Here's how the part is built. I have some questions about the finished solid (model axes, mm). Face numbers are marked on the shaded views. A direction names the side the tool comes from. Round coordinates to 2 decimals unless told otherwise and drop trailing zeros. Order: outer loops, then holes, each group sorted by start corner. A loop starts at its lowest first (then second) coordinate and runs counter-clockwise, first axis right, second up.
```python
from build123d import *


with BuildPart() as part:
    # Sketch1 → Revolve1 (revolve)
    with BuildSketch(Plane(origin=(0, 0, 0), x_dir=(-1, 0, 0), z_dir=(0, 0, -1)), mode=Mode.PRIVATE) as revolve1_sk:
        with BuildLine():
            Line((-1.5, -30), (0, -30))
            Line((0, -30), (0, 0))
            Line((0, 0), (-2.7, 0))
            ThreePointArc((-2.7, 0), (-2.95, -0.25), (-2.7, -0.5))
            Line((-2.7, -0.5), (-2.25, -2))
            Line((-2.25, -2), (-2, -2))
            Line((-2, -2), (-2, -29.5))
            Line((-2, -29.5), (-1.5, -30))
        make_face()
    revolve(revolve1_sk.sketch.rotate(Axis((0, -30, 0), (0, 1, 0)), 270), axis=Axis((0, -30, 0), (0, 1, 0)))


solid = part.part
```
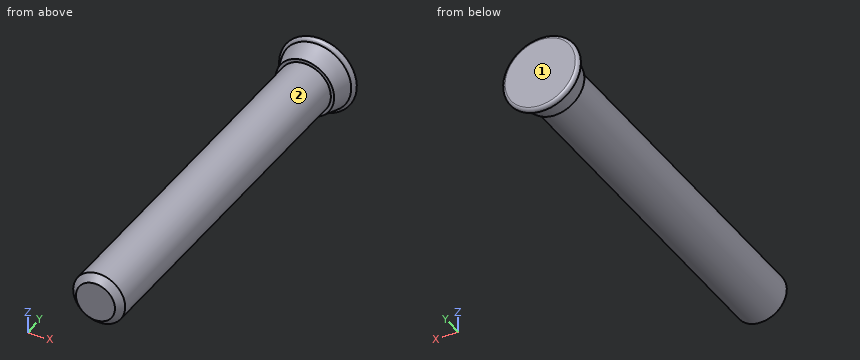
1. On a 3-axis mill with a long thin cutter (end or side, diameter ignored), from which of +Z, -Z, +X, -X, +Y, -Y can I reach the whole of each face in a straight line? I mean the marked faces 1 and 2. Say none if no direction works.
Evaluation:
face 1: +Z, -Z, +X, -X, +Y
face 2: -Y
2. I'm going to push flat-ended pins straight in: P1, Ø2, axis at y = -25.5, z = -1.5, coming from the -X side; P2, Ø1.5, axis at x = 1, y = -9.5, coming from the +Z side. Where does each tip first touch, or does it pass through?
Evaluation:
P1: stops at x = -1.94
P2: stops at z = 1.98
3. If we section it at B-B, the plane z = 0: Write out the boundary of the cut face in (x, y).
Evaluation:
outline: (-2.7, -0.5) - (-2.25, -2) - (-2, -2) - (-2, -29.5) - (-1.5, -30) - (1.5, -30) - (2, -29.5) - (2, -2) - (2.25, -2) - (2.7, -0.5) arc R0.25 ccw to (2.7, 0) - (-2.7, 0) arc R0.25 ccw to start
4. If we section it at A-A, the plane x = 0: Write out the boundary of the cut face in (y, z), and give its area (3 significant figures).
Evaluation:
outline: (-30, -1.5) - (-29.5, -2) - (-2, -2) - (-2, -2.25) - (-0.5, -2.7) arc R0.25 ccw to (0, -2.7) - (0, 2.7) arc R0.25 ccw to (-0.5, 2.7) - (-2, 2.25) - (-2, 2) - (-29.5, 2) - (-30, 1.5) - close
area: 122 mm2
5. I need wall thicknesses on probe 1 along X at (y, z) = (-17.5, -0.15); probe 2 along X at (y, z) = (-1.5, -1.8); probe 3 along Y at (x, z) = (1.55, -0.4). Which ranges of each line are inside material? Lowest first, please.
Evaluation:
probe 1: x = -1.99 to 1.99
probe 2: x = -1.59 to 1.59
probe 3: y = -29.9 to 0
6. If we section it at C-C, the plane y = -19.5: Write out the boundary of the cut face in (x, z).
Evaluation:
outline: circle Ø4 at (0, 0)
7. If we section it at D-D, the plane y = -1.75: Write out the boundary of the cut face in (x, z) (3 decimals).
Evaluation:
outline: circle Ø4.65 at (0, 0)
